Here's how the part is built. I have some questions about the finished solid (model axes, mm). Face numbers are marked on the shaded views. A direction names the side the tool comes from. Give positions to 0.01 mm unless a question says otherwise; leave off trailing zeros. Loops run counter-clockwise (first coordinate to the right, second up) from the corner with the lowest first, then second, coordinate; pieces in that order, holes last.
Q1. If we section it at D-D (y = 296.5): Please give me the cut outline in (x, z).
Q2. If we section it at C-C (z = -200): Please give me the cut outline in (x, y).
Q3. If we section it at A-A (x = 34): Please give me the cut outline in (y, z).
Q4. I need wall thicknesses on line 1 (Z direction, x = 57.5, y = 108.5); line 2 (X direction, y = 172.5, z = -205); line 3 (Z direction, x = 9, y = 95.5). Which ranges of each line are inside material? Lowest first, please.
Q5. For the marked faces 1, 2 and 3, which set-ups out of +Z, -Z, +X, -X, +Y, -Y let a thin tool reach every point of the face, with its end or its side?
Q6. If we section it at B-B (y = 68): Please give me the cut outline in (x, z).
Q7. Will these pins go through, and if not, where does the flat tip stop? P1, Ø1.5, axis at x = 21.5, y = 59.5, coming from the +Z side; P2, Ø6, axis at y = 277.5, z = 0.5, coming from the +X side; P3, Ø8, axis at x = 12, z = 95, coming from the +Y side.
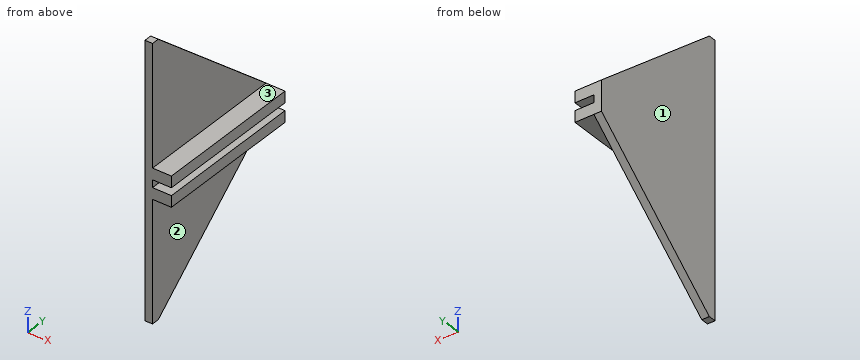
from build123d import *

# Parameters (mm, degrees)
BOSS_EXTRUDE1_DEPTH = 20
SKETCH3_W           = 30
SKETCH3_H           = 400
BOSS_EXTRUDE2_DEPTH = 50


with BuildPart() as part:
    # Sketch2 → Boss-Extrude1 (new body)
    with BuildSketch(Plane(origin=(0, 0, 0), x_dir=(0, 0, -1), z_dir=(1, 0, 0))):
        Polygon((-40, 400), (40, 400), (358.857859847, 20), (358.857859847, 0), (-358.857859847, 0), (-358.857859847, 20), align=None)
    extrude(amount=BOSS_EXTRUDE1_DEPTH)

    # Sketch3 → Boss-Extrude2 (add)
    with BuildSketch(Plane(origin=(20, 0, 0), x_dir=(0, 0, -1), z_dir=(1, 0, 0))):
        with Locations((-25, 200)):
            Rectangle(SKETCH3_W, SKETCH3_H)
        with Locations((25, 200)):
            Rectangle(SKETCH3_W, SKETCH3_H)
    extrude(amount=BOSS_EXTRUDE2_DEPTH)


solid = part.part
Check sheet entries:
1. outline: (0, -126.85) - (20, -126.85) - (20, -40) - (70, -40) - (70, -10) - (20, -10) - (20, 10) - (70, 10) - (70, 40) - (20, 40) - (20, 126.85) - (0, 126.85) - close
2. outline: (0, 0) - (20, 0) - (20, 209.32) - (0, 209.32) - close
3. outline: (0, -40) - (400, -40) - (400, -10) - (0, -10) - close; (0, 10) - (400, 10) - (400, 40) - (0, 40) - close
4. line 1: z = -40 to -10, 10 to 40
4. line 2: x = 0 to 20
4. line 3: z = -295.51 to 295.51
5. face 1: +Z, -Z, -X, +Y, -Y
5. face 2: -Z, +X, +Y, -Y
5. face 3: +Z, +X, +Y, -Y
6. outline: (0, -318.58) - (20, -318.58) - (20, -40) - (70, -40) - (70, -10) - (20, -10) - (20, 10) - (70, 10) - (70, 40) - (20, 40) - (20, 318.58) - (0, 318.58) - close
7. P1: stops at z = 40
7. P2: stops at x = 20
7. P3: stops at y = 339.22
